The listing builds one solid part. Answer for the finished solid, in the listing's coordinates (mm). A direction names the side the tool comes from. Give positions to 0.01 mm unless a question says otherwise; leave off trailing zeros. Order: outer loops, then holes, each group sorted by start corner. A loop starts at its lowest first (then second) coordinate and runs counter-clockwise, first axis right, second up. Notation, with made-up numbers: (-9, 2) - (18, 2) arc R26 cw to (18, 21) - close; hole circle Ø11 at (-8, 78). An arc over 180 degrees is marked (long way). Answer in a Markdown table with one row per item.
from build123d import *

# Parameters (mm, degrees)
CHANFREIN1_SIZE = 0.5
CHANFREIN2_SIZE = 0.5


with BuildPart() as part:
    # Sketch1 → Revolve1 (revolve)
    with BuildSketch(Plane.XY):
        Polygon((3.15, 0), (6, 0), (6, 2), (5.5, 2), (5, 2.5), (5, 7.75), (4, 7.75), (3.15, 1.75), align=None)
    revolve(axis=Axis((0, -36.960268038, 0), (0, 1, 0)))

    # Chanfrein1
    chanfrein1_edges = [part.edges().sort_by_distance(p)[0] for p in [
        (-6, 0, 0),
    ]]
    chamfer(chanfrein1_edges, length=CHANFREIN1_SIZE)

    # Chanfrein2
    chanfrein2_edges = [part.edges().sort_by_distance(p)[0] for p in [
        (-5, 7.75, 0),
    ]]
    chamfer(chanfrein2_edges, length=CHANFREIN2_SIZE)


solid = part.part
Item 1: Which of the six approach directions +Z, -Z, +X, -X, +Y, -Y give full straight-line access (tool end or side, diameter ignored) to faces 4 (the face through (-1.08, 4.91, 4.88)), 5 (the face through (-2.5, 0.863, 1.917))?
Answer block:
| item | result |
|---|---|
| face 4 | +Y |
| face 5 | +Y, -Y |
Item 2: Find section B-B on z = 0. Write down the section's boundary in (x, y), then the cut area to 3 significant figures.
Answer block:
| item | result |
|---|---|
| outline | (-6, 0.5) - (-5.5, 0) - (-3.15, 0) - (-3.15, 1.75) - (-4, 7.75) - (-4.5, 7.75) - (-5, 7.25) - (-5, 2.5) - (-5.5, 2) - (-6, 2) - close; (3.15, 0) - (5.5, 0) - (6, 0.5) - (6, 2) - (5.5, 2) - (5, 2.5) - (5, 7.25) - (4.5, 7.75) - (4, 7.75) - (3.15, 1.75) - close |
| area | 27.3 mm² |
Item 3: Find section C-C on y = 1.25. Write down the section's boundary in (x, z), then the cut area to 3 significant figures.
Answer block:
| item | result |
|---|---|
| outline | circle Ø12 at (0, 0); hole circle Ø6.3 at (0, 0) |
| area | 81.9 mm² |
Item 4: Consider line 1 (Z direction, x = 0, y = 1.1); line 2 (X direction, y = 3, z = 2.75). Determine where each line is inside the solid, lowest interval first.
Answer block:
| item | result |
|---|---|
| line 1 | -6 to -3.15, 3.15 to 6 |
| line 2 | -4.18 to -1.87, 1.87 to 4.18 |
Item 5: Determine the mould class of faces 1 (the face through (3, 2, 5)), 2 (the face through (-6, 1, 0)), 3 (the face through (-2.76, 4.04, 2.11)) for opening direction X: pulls with the +X half, pulls with the -X half, needs draft (parallel to the pull), parting line crosses it, or undercut.
Answer block:
| item | result |
|---|---|
| face 1 | needs draft |
| face 2 | parting line crosses it |
| face 3 | undercut |
Item 6: Each of these flat-tipped pins is pushed along its axis until it touches: P1, Ø3.5, axis at x = 2.5, z = 2.5, coming from the +Y side; P2, Ø2, axis at y = 6.5, z = 0.5, coming from the +X side; P3, Ø3, axis at x = -3, y = 2.5, coming from the +Z side; P4, Ø1.5, axis at x = 2, y = 6.5, coming from the +Z side. Where does it stop, or does it pass through?
Answer block:
| item | result |
|---|---|
| P1 | y = 7.75 |
| P2 | x = 5 |
| P3 | z = 5.79 |
| P4 | z = 4.84 |
Item 7: Find section A-A on x = 0. Write down the section's boundary in (y, z), then the cut area to 3 significant figures.
Answer block:
| item | result |
|---|---|
| outline | (0, -5.5) - (0.5, -6) - (2, -6) - (2, -5.5) - (2.5, -5) - (7.25, -5) - (7.75, -4.5) - (7.75, -4) - (1.75, -3.15) - (0, -3.15) - close; (0, 3.15) - (1.75, 3.15) - (7.75, 4) - (7.75, 4.5) - (7.25, 5) - (2.5, 5) - (2, 5.5) - (2, 6) - (0.5, 6) - (0, 5.5) - close |
| area | 27.3 mm² |
Item 8: Find section D-D on y = 3.5. Write down the section's boundary in (x, z).
Answer block:
| item | result |
|---|---|
| outline | circle Ø10 at (0, 0); hole circle Ø6.8 at (0, 0) |
